Can you work these out from the drawing? Everything is in mm from the part's minimum corner. A direction names the side the tool comes from. Round coordinates to 2 decimals unless told otherwise and drop trailing zeros. Write each loop counter-clockwise with the first axis right and the second up, starting at its lowest first coordinate (ties: lowest second). Pieces come first, ordered by that corner, then holes. Notation, with made-up numbers: (-35, -21.5) - (-20, -21.5) arc R18 cw to (-20, -5.5) - close; hole circle Ø3 at (68.5, 13.25). An arc over 180 degrees is marked (long way). One line per item, written item: value. Start each with the question number.
(1) I want a section at B-B on z = 20. List the corners of the cut face in (x, y) for me.
(2) I'm going to push flat-ended pins straight in: pin 1 Ø3 at (y, z) = (26, 11.5) entering from -X; pin 2 Ø19 at (x, z) = (20, 27.5) entering from +Y. Where does each tip first touch, or does it pass through?
(3) If I drill on L1, parallel to Z at x = 38.95, y = 15; L2, parallel to Y at x = 32, z = 18.5; L3, parallel to X at y = 12.5, z = 6, over which ranges is the centre line in solid material (lowest first)? Write a range as from..to.
(4) I want a section at D-D on y = 25. List the corners of the cut face in (x, z) for me.
(5) I want a section at A-A on y = 15. List the corners of the cut face in (x, z) for me.
(6) I want a section at C-C on z = 32.5. List the corners of the cut face in (x, y) for me.
(7) On a 3-axis mill with a long thin cutter (end or side, diameter ignored), from which of +Z, -Z, +X, -X, +Y, -Y can I reach the whole of each face in a straight line? I mean the marked faces 1 and 2. Say none if no direction works.
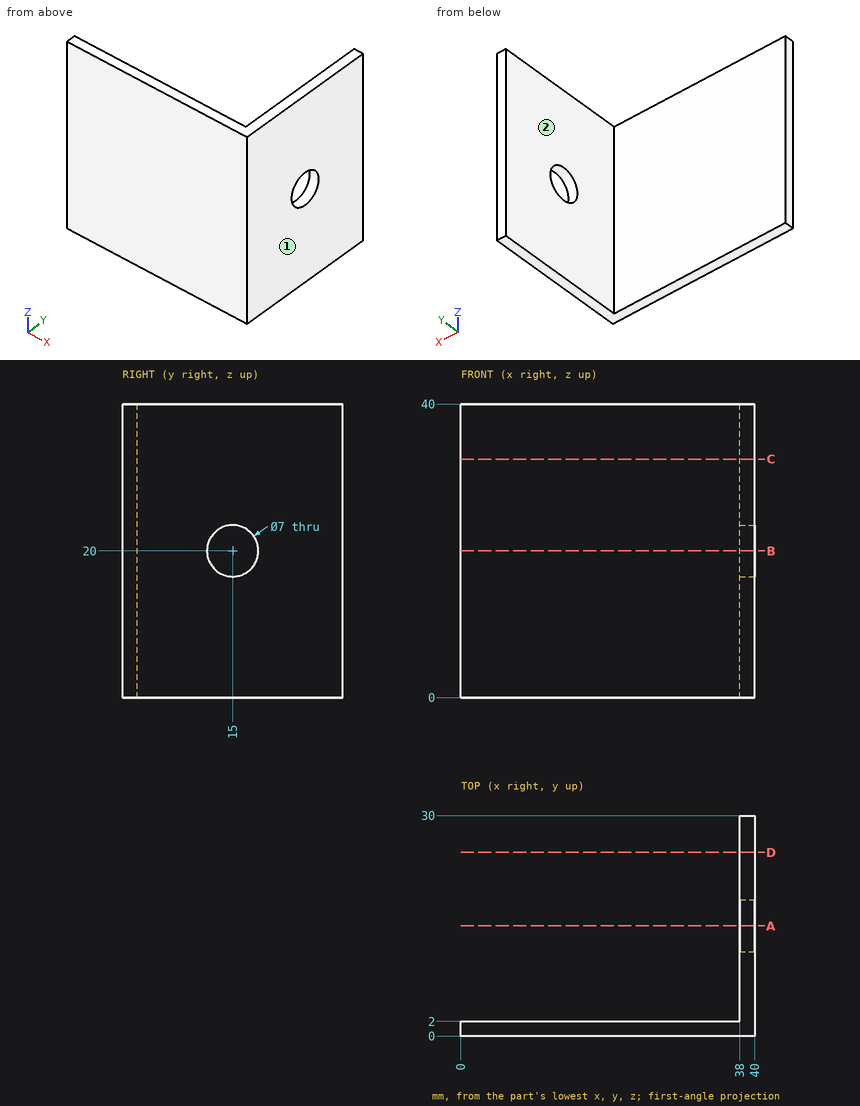
Established:
1. outline: (0, 0) - (40, 0) - (40, 11.5) - (38, 11.5) - (38, 2) - (0, 2) - close; (38, 18.5) - (40, 18.5) - (40, 30) - (38, 30) - close
2. pin 1: x = 38
2. pin 2: y = 2
3. L1: 0..16.5, 23.5..40
3. L2: 0..2
3. L3: 38..40
4. outline: (38, 0) - (40, 0) - (40, 40) - (38, 40) - close
5. outline: (38, 0) - (40, 0) - (40, 16.5) - (38, 16.5) - close; (38, 23.5) - (40, 23.5) - (40, 40) - (38, 40) - close
6. outline: (0, 0) - (40, 0) - (40, 30) - (38, 30) - (38, 2) - (0, 2) - close
7. face 1: +Z, -Z, +X, +Y, -Y
7. face 2: +Z, -Z, -X, +Y
